```python
from build123d import *

# Parameters (mm, degrees)
F0_W       = 234.745592
F0_H       = 312.781454
F1_DEPTH   = 199.39
F2_W       = 184.208318
F2_H       = 143.576262
F3_DEPTH   = 283.464
F4_W       = 181.309238
F4_H       = 140.677188
F5_DEPTH   = 248.158
F6_DEPTH   = 270.002
F7_W       = 181.055784
F7_H       = 164.668828
F8_DEPTH   = 273.05
F10_DEPTH  = 254
F11_W      = 44.579953
F11_H      = 312.781454
F12_DEPTH  = 25.4
F12_FACE_W = 44.579952
F12_FACE_H = 312.781454
F13_DEPTH  = 254


with BuildPart() as f1:
    # F0 (on Top) → F1 (new body)
    with BuildSketch(Plane.XY):
        Rectangle(F0_W, F0_H)
    extrude(amount=F1_DEPTH)

    # F2 (on face) → F3 (join)
    with BuildSketch(Plane.XZ.offset(156.390727)):
        with Locations((0, 86.327426)):
            Rectangle(F2_W, F2_H)
    extrude(amount=-F3_DEPTH)

    # F4 (on face) → F5 (join)
    with BuildSketch(Plane.XZ.offset(156.390727)):
        with Locations((0, 94.606221)):
            Rectangle(F4_W, F4_H)
    extrude(amount=-F5_DEPTH)

    # F4 (on face) → F6 (join)
    with BuildSketch(Plane.XZ.offset(156.390727)):
        with Locations((0, 94.606221)):
            Rectangle(F4_W, F4_H)
    extrude(amount=-F6_DEPTH)

    # F7 (on face) → F8 (cut)
    with BuildSketch(Plane.XZ.offset(156.390727)):
        with Locations((0, 98.565549)):
            Rectangle(F7_W, F7_H)
    extrude(amount=-F8_DEPTH, mode=Mode.SUBTRACT)

    # F9 (on face) → F10 (join)
    with BuildSketch(Plane(origin=(0, 0, 0), x_dir=(1, 0, 0), z_dir=(0, 0, -1))):
        Polygon((-78.603908, -156.390727), (-78.603908, -125.591993), (-78.603908, 125.591993), (-78.603908, 156.390727), (-117.372796, 156.390727), (-117.372796, -156.390727), align=None)
    extrude(amount=F10_DEPTH)

    # F11 (on face) → F12 (join)
    with BuildSketch(Plane(origin=(0, 0, 0), x_dir=(1, 0, 0), z_dir=(0, 0, -1))):
        with Locations((95.082819, 0)):
            Rectangle(F11_W, F11_H)
    extrude(amount=F12_DEPTH)

    # F12_face (on face) → F13 (join)
    with BuildSketch(Plane(origin=(95.082819, 0, -25.4), x_dir=(1, 0, 0), z_dir=(0, 0, -1))):
        Rectangle(F12_FACE_W, F12_FACE_H)
    extrude(amount=F13_DEPTH)


solid = f1.part
```
Check sheet for the modelled part. Datum: model origin and axes. Units: mm. A direction names the side the tool comes from. Round coordinates to 2 decimals unless told otherwise and drop trailing zeros. Loops run counter-clockwise (first coordinate to the right, second up) from the corner with the lowest first, then second, coordinate; pieces in that order, holes last. Notation, with made-up numbers: (10.5, 81) -> (65.5, 81) arc R25 ccw to (65.5, 117) -> close; hole circle Ø9 at (22, -36.75). An arc over 180 degrees is marked (long way). Write item = value, one per line. Start each with the question number.
1) Sectioned sample at A-A, the plane z = -13. Record the cut outline in (x, y).
2) Release check for a two-part mould opening along Z. For faces 4 (the flat face through (-1, 116.659, 100)), 5 (the flat face through (-117.373, -2, -24)), 6 (the flat face through (-98, -2, -254)), 7 (the flat face through (-1, -22, 16.231)) record: released by +Z, released by -Z, zero draft, split by the parting line, or undercut.
3) Sectioned sample at B-B, the plane x = -65. Record the cut outline in (y, z), plus the area to 3 significant figures.
4) Sectioned sample at C-C, the plane y = -71. Record the cut outline in (x, z).
5) Set-up check for faces 1 (the flat face through (1, -156.391, 14)), 2 (the flat face through (-4, 2, 0)), 3 (the flat face through (-1, -22, 180.9)): record each of +Z, -Z, +X, -X, +Y, -Y from which the full face is reachable in a straight line by a thin tool's end or side.
6) Thickness scan on probe 1 along Z at (x, y) = (22, -45); probe 2 along X at (y, z) = (40, -51); probe 3 along X at (y, z) = (-34, 162). Record the ranges inside material, lowest first.
7) Sectioned sample at D-D, the plane z = 106.5. Record the cut outline in (x, y).
8) Gauge pin test, flat ends, axial feed: pin 1 Ø19.5 at (x, y) = (-93.5, -36.5) entering from -Z; pin 2 Ø6 at (x, z) = (63, 37.5) entering from -Y. Record the tip position at first contact, or that the pin passes through.
Results are:
q1.outline = (-117.37, -156.39) -> (-78.6, -156.39) -> (-78.6, 156.39) -> (-117.37, 156.39) -> close; (72.79, -156.39) -> (117.37, -156.39) -> (117.37, 156.39) -> (72.79, 156.39) -> close
q2.face_4 = undercut
q2.face_5 = zero draft
q2.face_6 = released by -Z
q2.face_7 = undercut
q3.outline = (-156.39, 0) -> (156.39, 0) -> (156.39, 199.39) -> (-156.39, 199.39) -> (-156.39, 180.9) -> (116.66, 180.9) -> (116.66, 16.23) -> (-156.39, 16.23) -> close
q3.area = 17,400 mm^2
q4.outline = (-117.37, -254) -> (-78.6, -254) -> (-78.6, 0) -> (72.79, 0) -> (72.79, -279.4) -> (117.37, -279.4) -> (117.37, 199.39) -> (-117.37, 199.39) -> close; hole (-90.53, 16.23) -> (90.53, 16.23) -> (90.53, 180.9) -> (-90.53, 180.9) -> close
q5.face_1 = +Z, -Z, +X, -X, -Y
q5.face_2 = -Z, +Y, -Y
q5.face_3 = -Y
q6.probe_1 = 0 to 16.23, 180.9 to 199.39
q6.probe_2 = -117.37 to -78.6, 72.79 to 117.37
q6.probe_3 = -117.37 to -90.53, 90.53 to 117.37
q7.outline = (-117.37, -156.39) -> (-90.53, -156.39) -> (-90.53, 116.66) -> (90.53, 116.66) -> (90.53, -156.39) -> (117.37, -156.39) -> (117.37, 156.39) -> (-117.37, 156.39) -> close
q8.pin_1 = -254
q8.pin_2 = 116.66
